Geometry: final body of the model. Coordinates: model frame, mm. A direction names the side the tool comes from. Give positions to 0.01 mm unless a question says otherwise; leave off trailing zeros. Order: outer loops, then holes, each group sorted by start corner. A loop starts at its lowest first (then second) coordinate and runs counter-clockwise, first axis right, second up. Notation, with made-up numbers: (-14.75, -20) - (14.25, -20) arc R27 cw to (14.25, -2) - close; hole circle Ø1 at (20, 69.5). An arc over 180 degrees is marked (long way). Use one line per item in the form item = value.
from build123d import *

# Parameters (mm, degrees)
SKETCH2_W                       = 10
SKETCH2_H                       = 22.35
SKETCH2_R                       = 1.5
BOSS_EXTRUDE1_DEPTH             = 3.5
F_1_0MM_DOWEL_HOLE1_D           = 1
F_1_0MM_DOWEL_HOLE1_DEPTH       = 3
F_1_0MM_DOWEL_HOLE1_CSINK_D     = 1.05
F_1_0MM_DOWEL_HOLE1_CSINK_ANGLE = 90
F_1_0MM_DOWEL_HOLE1_TIP         = 0.30043031


with BuildPart() as part:
    # Sketch2 → Boss-Extrude1 (new body)
    with BuildSketch(Plane.XY):
        with Locations((0, -16.175)):
            Rectangle(SKETCH2_W, SKETCH2_H)
        with Locations((0, -7.3)):
            Circle(SKETCH2_R, mode=Mode.SUBTRACT)
        with Locations((0, -25.05)):
            Circle(SKETCH2_R, mode=Mode.SUBTRACT)
    extrude(amount=BOSS_EXTRUDE1_DEPTH)

    # Ø1.0mm Dowel Hole1
    with Locations(Plane(origin=(-4, -5, 1.7), x_dir=(1, 0, 0), z_dir=(0, 1, 0))):
        with Locations((0, 0), (8, 0)):
            CounterSinkHole(F_1_0MM_DOWEL_HOLE1_D / 2, F_1_0MM_DOWEL_HOLE1_CSINK_D / 2, depth=F_1_0MM_DOWEL_HOLE1_DEPTH, counter_sink_angle=F_1_0MM_DOWEL_HOLE1_CSINK_ANGLE)
            with Locations((0, 0, -(F_1_0MM_DOWEL_HOLE1_DEPTH + F_1_0MM_DOWEL_HOLE1_TIP / 2))):  # 118° drill point
                Cone(0, F_1_0MM_DOWEL_HOLE1_D / 2, F_1_0MM_DOWEL_HOLE1_TIP, mode=Mode.SUBTRACT)


solid = part.part
(1) Reachability of faces 5 (the face through (-5, -16, 2)), 6 (the face through (4.108, -6.533, 2.188)) from +Z, -Z, +X, -X, +Y, -Y: full face, straight path, thin tool, end or side. Return the list, or none.
Computed values:
face_5 = +Z, -Z, -X, +Y, -Y
face_6 = +Y
(2) Cut plane C-C on z = 3.1. Output: boundary loops of the cut face in (x, y), plus the area to 3 significant figures.
Computed values:
outline = (-5, -27.35) - (5, -27.35) - (5, -5) - (-5, -5) - close; hole circle Ø3 at (0, -25.05); hole circle Ø3 at (0, -7.3)
area = 209 mm²
(3) Ray query, line 1 along Y through (x, z) = (0, 1.8); line 2 along Z through (x, y) = (4, -6.25); line 3 along Y through (x, z) = (0.5, 0.2). Return the intervals inside material, ascending.
Computed values:
line_1 = -27.35 to -26.55, -23.55 to -8.8, -5.8 to -5
line_2 = 0 to 1.2, 2.2 to 3.5
line_3 = -27.35 to -26.46, -23.64 to -8.71, -5.89 to -5
(4) Cut plane A-A on y = -7.3. Output: boundary loops of the cut face in (x, z), plus the area to 3 significant figures.
Computed values:
outline = (-5, 0) - (-1.5, 0) - (-1.5, 3.5) - (-5, 3.5) - close; (1.5, 0) - (5, 0) - (5, 3.5) - (1.5, 3.5) - close; hole circle Ø1 at (-4, 1.7); hole circle Ø1 at (4, 1.7)
area = 22.9 mm²
(5) Contact query for a flat-ended pin moving along its axis: pin 1 Ø1.5 at (x, y) = (1, -24) entering from -Z. Output: stop coordinate, or through.
Computed values:
pin_1 = 0
(6) Pull-direction query (Y, two-part tool) for faces 1 (the face through (5, -16, 2)), 2 (the face through (-0.325, -8.764, 1.726)), 3 (the face through (0, -5, 2)), 4 (the face through (-0.195, -23.563, 1.726)); classes: released by +Y, released by -Y, zero draft, split by the parting line, or undercut.
Computed values:
face_1 = zero draft
face_2 = undercut
face_3 = released by +Y
face_4 = undercut
(7) Cut plane B-B on y = -25.05. Output: boundary loops of the cut face in (x, z), plus the area to 3 significant figures.
Computed values:
outline = (-5, 0) - (-1.5, 0) - (-1.5, 3.5) - (-5, 3.5) - close; (1.5, 0) - (5, 0) - (5, 3.5) - (1.5, 3.5) - close
area = 24.5 mm²
